Here's how the part is built. I have some questions about the finished solid (model axes, mm). A direction names the side the tool comes from. Give positions to 0.01 mm unless a question says otherwise; leave off trailing zeros. Loops run counter-clockwise (first coordinate to the right, second up) from the corner with the lowest first, then second, coordinate; pieces in that order, holes last.
Q1. I'm going to push flat-ended pins straight in: P1, Ø10, axis at x = 27, y = -40.5, coming from the -Z side; P2, Ø4, axis at x = -9, z = 66, coming from the -Y side. Where does each tip first touch, or does it pass through?
Q2. Suppose I cut it at D-D (z = 47). List the corners of the cut face in (x, y) for me, and give its area (3 significant figures).
Q3. For faces 1 (the face through (92.71, 8.06, 2.67)), 2 (the face through (-24.34, 8.06, 2.67)), 3 (the face through (35, 2.566, 37)), 4 (the face through (94.631, 6, 3)), 5 (the face through (-26.369, 6, 3)), which set-ups out of +Z, -Z, +X, -X, +Y, -Y let a thin tool reach every point of the face, with its end or its side?
Q4. I need wall thicknesses on probe 1 along Y at (x, z) = (10, 17); probe 2 along Z at (x, y) = (69, -30.5); probe 3 along X at (y, z) = (5, 34). Which ranges of each line are inside material? Lowest first, please.
Q5. Suppose I cut it at C-C (y = -14.5). List the corners of the cut face in (x, z) for me.
Q6. Suppose I cut it at B-B (x = -10.5). List the corners of the cut face in (y, z) for me, and give its area (3 significant figures).
Q7. Suppose I cut it at A-A (z = 3). List the corners of the cut face in (x, y) for me.
```python
from build123d import *

# Parameters (mm, degrees)
SKETCH1_W                = 113.11
SKETCH1_H                = 5
BOSS_EXTRUDE1_DEPTH      = 80
SKETCH2_W                = 113.11
SKETCH2_H                = 4
BOSS_EXTRUDE3_DEPTH      = 53.07
BOSS_EXTRUDE4_DEPTH      = 4
BOSS_EXTRUDE4_DEPTH_BACK = 117
SKETCH3_R                = 2.5
SKETCH4_W                = 113.11
SKETCH4_H                = 1.014466344
BOSS_EXTRUDE5_DEPTH      = 79
SKETCH5_W                = 0.8
SKETCH5_H                = 62.100076999
CUT_EXTRUDE2_DEPTH       = 224


with BuildPart() as part:
    # Sketch1 → Boss-Extrude1 (new body)
    with BuildSketch(Plane.XY):
        with Locations((34.185736393, 6.080576307)):
            Rectangle(SKETCH1_W, SKETCH1_H)
    extrude(amount=BOSS_EXTRUDE1_DEPTH)

    # Sketch2 → Boss-Extrude3 (add)
    with BuildSketch(Plane.XZ.offset(-3.580576307)):
        with Locations((34.185736393, 78)):
            Rectangle(SKETCH2_W, SKETCH2_H)
    extrude(amount=BOSS_EXTRUDE3_DEPTH)

    # Sketch3 → Boss-Extrude4 (add, two sides: drawn at the far end of the back side and taken through both)
    with BuildSketch(Plane.ZY.offset(22.369263607).offset(-BOSS_EXTRUDE4_DEPTH_BACK)):
        with Locations((3, 5.580576307)):
            Circle(SKETCH3_R)
    extrude(amount=BOSS_EXTRUDE4_DEPTH + BOSS_EXTRUDE4_DEPTH_BACK)

    # Sketch4 → Boss-Extrude5 (add)
    with BuildSketch(Plane(origin=(0, 0, 0), x_dir=(-1, 0, 0), z_dir=(0, 0, -1))):
        with Locations((-34.185736393, 3.073343135)):
            Rectangle(SKETCH4_W, SKETCH4_H)
    extrude(amount=-BOSS_EXTRUDE5_DEPTH)

    # Sketch5 → Cut-Extrude2 (cut)
    with BuildSketch(Plane.ZY.offset(22.369263607)):
        with Locations((79.6, -22.469462192)):
            Rectangle(SKETCH5_W, SKETCH5_H)
    extrude(amount=-CUT_EXTRUDE2_DEPTH, mode=Mode.SUBTRACT)


solid = part.part
```
Solutions:
1. P1: stops at z = 76
1. P2: stops at y = 2.57
2. outline: (-22.37, 2.57) - (90.74, 2.57) - (90.74, 8.58) - (-22.37, 8.58) - close
2. area: 680 mm2
3. face 1: +X
3. face 2: -X
3. face 3: -Z, +X, -X, -Y
3. face 4: +Z, -Z, +X, +Y, -Y
3. face 5: +Z, -Z, -X, +Y, -Y
4. probe 1: y = 2.57 to 8.58
4. probe 2: z = 76 to 79.2
4. probe 3: x = -22.37 to 90.74
5. outline: (-22.37, 76) - (90.74, 76) - (90.74, 79.2) - (-22.37, 79.2) - close
6. outline: (-49.49, 76) - (2.57, 76) - (2.57, 0) - (8.58, 0) - (8.58, 79.2) - (-49.49, 79.2) - close
6. area: 643 mm2
7. outline: (-26.37, 3.08) - (-22.37, 3.08) - (-22.37, 2.57) - (90.74, 2.57) - (90.74, 3.08) - (94.63, 3.08) - (94.63, 8.08) - (90.74, 8.08) - (90.74, 8.58) - (-22.37, 8.58) - (-22.37, 8.08) - (-26.37, 8.08) - close
